Autodesk Inventor part; units mm, degrees
ref_plane "YZ Plane" through (0, 0, 0) normal (1, 0, 0) x (0, 1, 0)
ref_plane "XZ Plane" through (0, 0, 0) normal (0, 1, 0) x (-1, 0, 0)
ref_plane "XY Plane" through (0, 0, 0) normal (0, 0, 1) x (1, 0, 0)
sketch "スケッチ1" plane through (0, 0, 0) normal (0, 0, 1) x (1, 0, 0)
  circle A0 centre (0, 9) radius 7.75
  line L0 (10.75, 0) -> (-58.5, 0)
  line L1 (-58.5, 0) -> (-58.5, 1.25)
  line L2 (-58.5, 1.25) -> (10.75, 1.25)
  line L3 (10.75, 1.25) -> (10.75, 0)
  circle A1 centre (0, 9) radius 10.75
  line L4 (10.75, 1.25) -> (10.75, 15.8822)
  circle A2 centre (-32, 9) radius 2.5
  circle A3 centre (-39, 9) radius 2.5
  circle A4 centre (-25, 9) radius 3.5
  circle A5 centre (-46, 9) radius 2.5
  circle A6 centre (-53, 9) radius 2.5
  circle A7 centre (-53, 9) radius 5.5
  line L5 (-58.5, 1.25) -> (-58.5, 21.0928)
  line L6 (-61.1769, 14.5) -> (16.6826, 14.5)
  point P0 (0, 0)
  point P1 (-9.2365, 14.5)
  point P2 (-58.5, 14.5)
  point P3 (10.75, 14.5)
  point P4 (9.2365, 14.5)
  point P5 (10.75, 9)
  point P6 (5.879, 0)
  point P7 (-5.879, 0)
  dimension "d0" = 15.5
  dimension "d1" = 3
  dimension "d2" = 5
  dimension "d3" = 5
  dimension "d4" = 7
  dimension "d5" = 5
  dimension "d7" = 7
  dimension "d8" = 7
  dimension "d9" = 25
  dimension "d10" = 7
  dimension "d11" = 5
  dimension "d12" = 7
  dimension "d13" = 3
  dimension "d16" = 9
extrude "押し出し1" add sketch "スケッチ1" along normal blind 20 contours A0 L6 A1 L2 | A0 L6 A1 | L2 A1 L6 A0 | L2 A1 L0 | L6 L4 A1 | A1 L0 L1 L2 | L2 L5 A7 A5 L6 A1 | A1 L4 L2 | L2 L3 L0 A1 | A7 A5 | A7 L5 L6 picked at (-49.0972, 10.8197)
sketch "スケッチ3" plane through (0, 0, 20) normal (0, 0, 1) x (1, 0, 0)
  line L0 (-9.2365, 14.5) -> (-58.5, 14.5)
  line L1 (-58.5, 14.5) -> (-58.5, 0)
  line L2 (-58.5, 0) -> (10.75, 0)
  arc A0 (9.2365, 14.5) -> (-9.2365, 14.5) centre (0, 9) ccw
  circle A1 centre (0, 9) radius 7.75
  circle A2 centre (-53, 9) radius 2.5
  circle A3 centre (-25, 9) radius 3.5
  circle A4 centre (-39, 9) radius 2.5
  circle A5 centre (-32, 9) radius 2.5
  circle A6 centre (-46, 9) radius 2.5
  line L3 (-58.5, 14.5) -> (-58.5, 0)
  line L4 (-58.5, 0) -> (-68.5, 0)
  line L5 (-68.5, 0) -> (-68.5, 14.5)
  line L6 (-68.5, 14.5) -> (-58.5, 14.5)
  line L7 (-58.5, 14.5) -> (-58.5, 0)
  line L8 (10.75, -0.0065) -> (20.75, -0.0065)
  line L9 (20.75, -0.0065) -> (20.75, 14.5)
  line L10 (20.75, 14.5) -> (10.75, 14.5)
  line L11 (10.75, 14.5) -> (10.75, -0.0065)
  line L12 (10.75, 0) -> (10.75, 14.5)
  line L13 (10.75, 14.5) -> (9.2365, 14.5)
  point P0 (0, 0)
  dimension "d17" = 10
  dimension "d18" = 10
extrude "押し出し2" add sketch "スケッチ3" against normal up to surface (20 mm away) contours L1 L4 L5 L6 | L10 L9 L8 L11
sketch "スケッチ4" plane through (0, 0, 20) normal (0, 0, 1) x (1, 0, 0)
  line L0 (-9.2365, 14.5) -> (-68.5, 14.5)
  line L1 (-68.5, 14.5) -> (-68.5, 0)
  line L2 (-68.5, 0) -> (10.75, 0)
  line L3 (20.75, -0.0065) -> (20.75, 14.5)
  line L4 (20.75, 14.5) -> (9.2365, 14.5)
  arc A0 (9.2365, 14.5) -> (-9.2365, 14.5) centre (0, 9) ccw
  circle A1 centre (0, 9) radius 7.75
  circle A2 centre (-53, 9) radius 2.5
  circle A3 centre (-25, 9) radius 3.5
  circle A4 centre (-39, 9) radius 2.5
  circle A5 centre (-32, 9) radius 2.5
  circle A6 centre (-46, 9) radius 2.5
  line L5 (-68.5, 0) -> (-68.5, 14.5)
  line L6 (-68.5, 9) -> (20.75, 9)
  line L7 (20.75, 9) -> (20.75, 30.4065)
  line L8 (20.75, 30.4065) -> (-68.5, 30.4065)
  line L9 (-68.5, 30.4065) -> (-68.5, 9)
  line L10 (10.75, 0) -> (10.75, -0.0065)
  line L11 (10.75, -0.0065) -> (20.75, -0.0065)
  point P0 (0, 0)
  point P1 (-55.5, 9)
  point P2 (-40.5, 9)
  point P3 (-48.5, 9)
  point P4 (-33.5, 9)
  point P5 (-41.5, 9)
  point P6 (-26.5, 9)
  point P7 (-34.5, 9)
  point P8 (-19.5, 9)
  point P9 (-18.5, 9)
  point P10 (-21.5, 9)
  point P11 (7.75, 9)
  point P12 (7.75, 9)
  point P13 (10.75, 9)
  point P14 (-21.5, 9)
  point P15 (-28.5, 9)
  point P16 (-29.5, 9)
  point P17 (-29.5, 9)
  point P18 (-36.5, 9)
  point P19 (-36.5, 9)
  point P20 (-43.5, 9)
  point P21 (-43.5, 9)
  point P22 (-50.5, 9)
  point P23 (-50.5, 9)
  point P24 (-68.5, 14.5065)
  point P25 (20.75, 14.5)
  point P26 (-68.5, 14.5)
  point P27 (20.75, 14.5)
extrude "押し出し3" cut sketch "スケッチ4" against normal through all contours A0 L4 L3 L6 A1 A3 A5 A4 A6 A2 L1 L0 | L0 L9 L8 L7 L4 A0 | A2 L6 | L6 A1 | A6 L6 | L6 A3 | A4 L6 | L6 A5 picked at (-52.3762, 9.5526) picked at (1.4675, 11.126) picked at (-45.3762, 9.5526) picked at (-24.5863, 10.0909) picked at (-38.3762, 9.5526) picked at (-32.7192, 9.9399)
sketch "スケッチ6" plane through (7.75, 9, 20) normal (0, 1, 0) x (1, 0, 0)
  line L0 (0, 0) -> (0, 20)
  line L1 (13, 0) -> (0, 0)
  line L2 (13, 20) -> (13, 0)
  line L3 (-29.25, 0) -> (-29.25, 20)
  line L4 (-15.5, 0) -> (-29.25, 0)
  line L5 (-15.5, 20) -> (-15.5, 0)
  line L6 (-63.25, 20) -> (-63.25, 0)
  line L7 (-76.25, 0) -> (-76.25, 20)
  line L8 (-63.25, 0) -> (-76.25, 0)
  line L9 (-76.25, 20) -> (-63.25, 20)
  line L10 (-29.25, 20) -> (-15.5, 20)
  line L11 (0, 20) -> (13, 20)
  point P0 (-7.75, 20)
  point P1 (8, 10)
  point P2 (-23.5, 10)
  point P3 (-71.25, 10)
  dimension "d33" = 10
  dimension "d34" = 5
  dimension "d35" = 5
  dimension "d36" = 15.75
hole "穴2" at (15.75, 9, 10) at (-15.75, 9, 10) at (-63.5, 9, 10) direction (0, -1, 0) diameter 4.3 end through all
chamfer "面取り1" distance 2 angle 45 4 edges at (20.75, 4.4968, 0) (20.75, 4.4968, 20) (-68.5, 4.5, 0) (-68.5, 4.5, 20)
properties part number "C_Unit_Cable_Holder_B"
For this review, take the finished solid that the model builds, in its own axes (mm). Round coordinates to 2 decimals unless told otherwise and drop trailing zeros. Write each loop counter-clockwise with the first axis right and the second up, starting at its lowest first coordinate (ties: lowest second). Pieces come first, ordered by that corner, then holes. Notation, with made-up numbers: (41.25, 18) -> (87.25, 18) arc R25 cw to (87.25, 30) -> close; hole circle Ø1 at (-3.75, 72). An arc over 180 degrees is marked (long way). One line per question, with ' | ' between items. Start each with the question number.
1) Mouldability with a two-part tool opening along Z and no side actions: class faces 1 (the cylindrical face through (-52.9, 6.5, 9.9)), 2 (the cylindrical face through (17.85, 4.43, 9.53)), 3 (the flat face through (-67.5, 4.6, 1)) as +Z half, -Z half, draft (parallel to the pull), parting line (faces both ways), or undercut.
2) Add section C-C (y = 3.5). Write out the cut boundary in (x, z).
3) Wall thickness on line 1 along Z through (x, y) = (15.75, 6); line 2 along X through (y, z) = (4, 10); line 3 along X through (y, z) = (3, 10): over which ranges is each line inside the solid? List them lowest first.
4) Add section B-B (x = -15.75). Write out the cut boundary in (y, z), and give its area (3 significant figures).
5) For pin 1 Ø5.5 at (x, z) = (-15.75, 10) entering from -Y, flat-tipped, find the tip position at first contact; note if it passes through.
6) Add section A-A (z = 10). Count the separate pieces of the cut face and the enclosed holes in it, and give its area (3 significant figures).
Reported:
1) face 1: draft | face 2: undercut | face 3: -Z half
2) outline: (-68.5, 2) -> (-66.5, 0) -> (-5.46, 0) -> (-5.46, 20) -> (-66.5, 20) -> (-68.5, 18) -> close; (5.46, 0) -> (18.75, 0) -> (20.75, 2) -> (20.75, 18) -> (18.75, 20) -> (5.46, 20) -> close; hole circle Ø4.3 at (-63.5, 10); hole circle Ø4.3 at (-15.75, 10); hole circle Ø4.3 at (15.75, 10)
3) line 1: z = 0 to 7.85, 12.15 to 20 | line 2: x = -68.5 to -65.65, -61.35 to -17.9, -13.6 to -5.92, 5.92 to 13.6, 17.9 to 20.75 | line 3: x = -68.5 to -65.65, -61.35 to -17.9, -13.6 to -4.91, 4.91 to 13.6, 17.9 to 20.75
4) outline: (0, 0) -> (9, 0) -> (9, 7.85) -> (0, 7.85) -> close; (0, 12.15) -> (9, 12.15) -> (9, 20) -> (0, 20) -> close | area: 141 mm²
5) pin 1: stops at y = 0
6) separate pieces: 4 | enclosed holes: 0 | area: 534 mm²
